Autodesk Inventor part; units mm, degrees
ref_plane "工作平面1" through (3.4, 0, 0) normal (1, 0, 0) x (0, 1, 0)
ref_plane "XZ Plane" through (0, 0, 0) normal (0, 1, 0) x (-1, 0, 0)
ref_plane "XY Plane" through (0, 0, 0) normal (0, 0, 1) x (1, 0, 0)
sketch "草圖1" plane through (0, 0, 0) normal (0, 0, 1) x (1, 0, 0)
  circle A0 centre (0, 0) radius 3.4
  dimension "d0" = 6.8
extrude "擠出1" add sketch "草圖1" along normal blind 6.5
sketch "草圖2" plane through (0, 0, 6.5) normal (0, 0, 1) x (1, 0, 0)
  circle A0 centre (0, 0) radius 1.55
  dimension "d3" = 3.1
extrude "擠出2" cut sketch "草圖2" against normal up to surface (6.5 mm away)
ref_plane "工作平面1" through (3.4, 0, 0) normal (1, 0, 0) x (0, 1, 0)
sketch "草圖3" plane through (3.4, 0, 0) normal (1, 0, 0) x (0, 1, 0)
  circle A0 centre (0, 1.5) radius 1.5
  line L0 (0, -1.3) -> (0, 7.8)
  line L1 (3.4, 0) -> (-3.4, 0)
  point P0 (0, 0)
  dimension "d6" = 3
extrude "擠出3" cut sketch "草圖3" against normal up to surface
sketch "草圖4" plane through (0, 0, 6.5) normal (0, 0, 1) x (1, 0, 0)
  circle A0 centre (0, 2.5) radius 0.9
  circle A1 centre (0, -2.5) radius 0.9
  line L0 (-0.7895, 2.932) -> (-2.3938, 0)
  line L1 (-2.3938, 0) -> (-0.7895, -2.932)
  line L2 (0.7895, 2.932) -> (2.3938, 0)
  line L3 (2.3938, 0) -> (0.7895, -2.932)
  circle A2 centre (-1.5389, 0) radius 0.75
  line L4 (3.4, 0) -> (1.55, 0)
  circle A3 centre (1.5389, 0) radius 0.75
  line L5 (0, -4.76) -> (0, 4.76)
  circle A4 centre (0, 0) radius 3.4
  circle A5 centre (0, 0) radius 2.1
  point P0 (0, 3.4)
  point P1 (2.1968, 0.36)
  point P2 (2.1968, -0.36)
  point P3 (0, -3.4)
  point P4 (-2.1968, -0.36)
  point P5 (-2.1968, 0.36)
  dimension "d10" = 1.8
  dimension "d13" = 1.5
  dimension "d16" = 4.2
extrude "擠出4" cut sketch "草圖4" against normal blind 3 contours A0 A4 L4 L2 | A0 L0 L1 A1 A4 | A4 A1 L3 L4 | L2 L4 A3 | L3 A3 L4 | A2 L1 L0
sketch "草圖5" plane through (0, 0, 6.5) normal (0, 0, 1) x (1, 0, 0)
  arc A0 (-0.7895, -2.932) -> (0.7895, -2.932) centre (0, -2.5) ccw
  line L0 (0.7895, -2.932) -> (2.1968, -0.36)
  arc A1 (2.1968, -0.36) -> (2.1968, 0.36) centre (1.5389, 0) ccw
  line L1 (2.1968, 0.36) -> (0.7895, 2.932)
  arc A2 (0.7895, 2.932) -> (-0.7895, 2.932) centre (0, 2.5) ccw
  line L2 (-0.7895, 2.932) -> (-2.1968, 0.36)
  arc A3 (-2.1968, 0.36) -> (-2.1968, -0.36) centre (-1.5389, 0) ccw
  line L3 (-2.1968, -0.36) -> (-0.7895, -2.932)
  circle A4 centre (0, 0) radius 1.55
extrude "擠出5" add sketch "草圖5" along normal blind 3
fillet "圓角1" radius 0.2 1 edges at (-1.55, 0, 9.5)
properties part number "Coupling_0519"
The model under review builds one solid part; all positions refer to its coordinate system, in mm. A direction names the side the tool comes from. Round coordinates to 2 decimals unless told otherwise and drop trailing zeros. Loops run counter-clockwise (first coordinate to the right, second up) from the corner with the lowest first, then second, coordinate; pieces in that order, holes last. Notation, with made-up numbers: (20.5, -13.5) - (65.5, -13.5) arc R13 ccw to (65.5, 6.5) - close; hole circle Ø4 at (56, -3.75). An arc over 180 degrees is marked (long way). Use CSV: the item, a comma, the result in double quotes.
(1) Machinability: for faces 4 (the flat face through (3, 0, 3.5)), 5 (the cylindrical face through (0, -3.4, 8)), 6 (the cylindrical face through (0, 3.4, 5)), which of the approach directions +Z, -Z, +X, -X, +Y, -Y give a long, thin tool a straight path to every point of the face, cutting with its end or side? Answer none if there is none.
Working result:
face 4,"+Z, +X"
face 5,"+Z, -Y"
face 6,"+Z, +Y"
(2) Take a section at A-A, the plane z = 8.25. Give the boundary of the cut face in (x, y).
Working result:
outline,"(-2.2, -0.36) - (-0.79, -2.93) arc R0.9 ccw to (0.79, -2.93) - (2.2, -0.36) arc R0.75 ccw to (2.2, 0.36) - (0.79, 2.93) arc R0.9 ccw to (-0.79, 2.93) - (-2.2, 0.36) arc R0.75 ccw to start; hole circle Ø3.1 at (0, 0)"
(3) For line 1 (Y direction, x = 0, z = 5); line 2 (Y direction, x = 1, z = 6.5); line 3 (X direction, y = -0.25, z = 6), list the stretches that pass through material, from the lowest coordinate up.
Working result:
line 1,"y = -3.4 to -1.55, 1.55 to 3.4"
line 2,"y = -2.55 to -1.18, 1.18 to 2.55"
line 3,"x = -2.25 to -1.53, 1.53 to 2.25"
(4) Take a section at B-B, the plane y = -2.5. Give the boundary of the cut face in (x, z).
Working result:
outline,"(-2.3, 0) - (2.3, 0) - (2.3, 3.5) - (1.03, 3.5) - (1.03, 9.5) - (-1.03, 9.5) - (-1.03, 3.5) - (-2.3, 3.5) - close"
(5) The part is to be moulded in two halves that separate along X. For faces 1 (the cylindrical face through (0, 3.4, 8)), 2 (the cylindrical face through (-1.55, 0.07, 4.72)), 3 (the flat face through (-1, 2, 9.5)), say which applies: pulls with the +X half, pulls with the -X half, needs draft (parallel to the pull), parting line crosses it, or undercut.
Working result:
face 1,"parting line crosses it"
face 2,"undercut"
face 3,"needs draft"
(6) Take a section at C-C, the plane z = 1.5. Give the boundary of the cut face in (x, y).
Working result:
outline,"(0.39, -1.5) arc R1.55 cw (long way) to (0.39, 1.5) - (3.05, 1.5) arc R3.4 ccw (long way) to (3.05, -1.5) - close"
(7) Clearance check with flat-ended pins moving along their axes: P1, Ø2, axis at x = 1.5, z = 6, coming from the -Y side; P2, Ø2, axis at y = -1.5, z = 7.5, coming from the -X side; P3, Ø1.5, axis at x = -2.5, z = 8, coming from the +Y side. State where each tip first meets the part, or that it passes through.
Working result:
P1,"stops at y = -3.25"
P2,"stops at x = -2.12"
P3,"stops at y = 1.18"
